Verification items for this drawing (mm, ordinates from the low corner). A direction names the side the tool comes from. Give positions to 0.01 mm unless a question says otherwise; leave off trailing zeros. Loops run counter-clockwise (first coordinate to the right, second up) from the corner with the lowest first, then second, coordinate; pieces in that order, holes last. Notation, with made-up numbers: (-27, -38.75) - (-7, -38.75) arc R21 cw to (-7, -20.75) - close; hole circle Ø11 at (83, 32). An arc over 180 degrees is marked (long way). Write item = value, one per line. Start each with the question number.
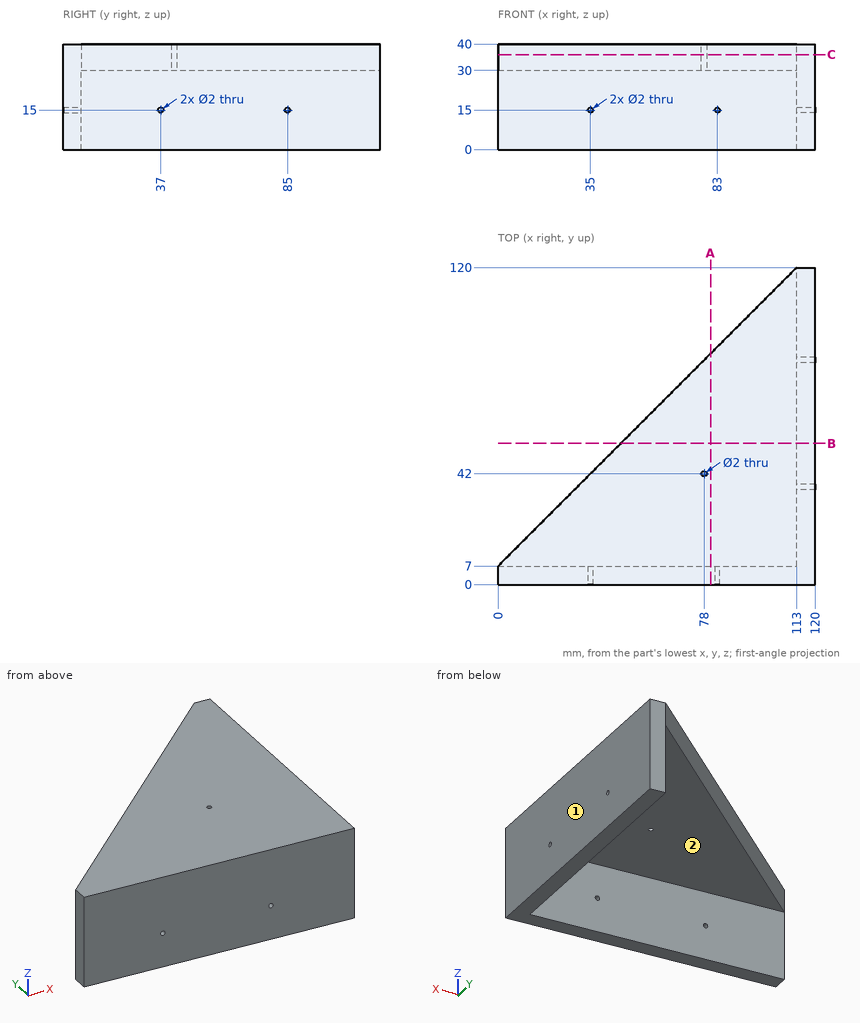
1) Tool access check on the marked faces 1 and 2. Record the directions out of +Z, -Z, +X, -X, +Y, -Y that give a thin tool (end or side, any length) a straight path to the whole face; none if there is none.
2) Gauge pin test, flat ends, axial feed: P1, Ø1, axis at y = 68.5, z = 34, coming from the -X side; P2, Ø15, axis at x = 47.5, z = 10.5, coming from the +Y side; P3, Ø3, axis at x = 78, y = 42, coming from the -Z side. Record the tip position at first contact, or that the pin passes through.
3) Material ranges on line 1 along Y through (x, z) = (118.5, 15); line 2 along Z through (x, y) = (83, 2.75); line 3 along Z through (x, y) = (108, 90), recorded low to high.
4) Cross-section at A-A on x = 80.5. Enter the section's corners in (y, z), and give its area (4 significant figures).
5) Cross-section at B-B on y = 53.5. Enter the section's corners in (x, z), and give its area (3 significant figures).
6) Cross-section at C-C on z = 36. Enter the section's corners in (x, y), and give its area (3 significant figures).
Checked values:
q1.face_1 = +Z, -Z, +X, +Y, -Y
q1.face_2 = -Z, -X, +Y
q2.P1 = 61
q2.P2 = 7
q2.P3 = 30
q3.line_1 = 0 to 36, 38 to 84, 86 to 120
q3.line_2 = 0 to 14, 16 to 40
q3.line_3 = 30 to 40
q4.outline = (0, 0) - (7, 0) - (7, 30) - (87.5, 30) - (87.5, 40) - (0, 40) - close
q4.area = 1,085 mm²
q5.outline = (46.5, 30) - (113, 30) - (113, 0) - (120, 0) - (120, 40) - (46.5, 40) - close
q5.area = 945 mm²
q6.outline = (0, 0) - (120, 0) - (120, 120) - (113, 120) - (0, 7) - close; hole circle Ø2 at (78, 42)
q6.area = 8,010 mm²
